Input: dimensioned drawing with shaded views. Units: mm. Origin: part minimum x, y, z. A direction names the side the tool comes from. Give positions to 0.01 mm unless a question says otherwise; leave off trailing zeros. Order: outer loops, then holes, each group sorted by start corner. A loop starts at its lowest first (then second) coordinate and runs counter-clockwise, first axis right, second up. Notation, with made-up numbers: M -0.75,88 L 7.25,88 A4 ccw 7.25,94 Z; hole C -27.5,0 d2. An arc over 180 degrees is marked long. Answer in a Markdown table with one row per item. Add a question column.
(1) Set-up query: the marked faces 4 and 5. Return all of +Z, -Z, +X, -X, +Y, -Y with unobstructed straight access to the full face (end or side cutting, diameter ignored); none if empty.
(2) Section query D-D, the plane y = 5. Return loops of the section in (x, z), plus the area to 3 significant figures.
(3) Section query A-A, the plane y = 29. Return loops of the section in (x, z).
(4) Section query B-B, the plane x = 11. Return loops of the section in (y, z).
(5) Material intervals for line 1 along X through (y, z) = (30.5, 7.5); line 2 along Z through (x, y) = (27, 51); line 3 along X through (y, z) = (46, 8), sorted ascending.
(6) Mould query, pull axis Y, two halves, no side actions, for the marked faces 1, 2 and 3. Classes: pulls with the +Y half, pulls with the -Y half, needs draft (parallel to the pull), parting line crosses it, or undercut.
(7) Section query C-C, the plane z = 8.25. Return loops of the section in (x, y) (3 decimals), plus the area to 3 significant figures.
(8) Pin query (flat end, axial travel): P1, Ø4, axis at y = 24, z = 5, coming from the +X side; P2, Ø2, axis at x = 35.5, y = 15, coming from the +Z side; P3, Ø1, axis at y = 22, z = 5.5, coming from the +X side; P4, Ø1.5, axis at x = 28.5, y = 46.5, coming from the -Z side. Return the tip coordinate at first contact, or that it passes through.
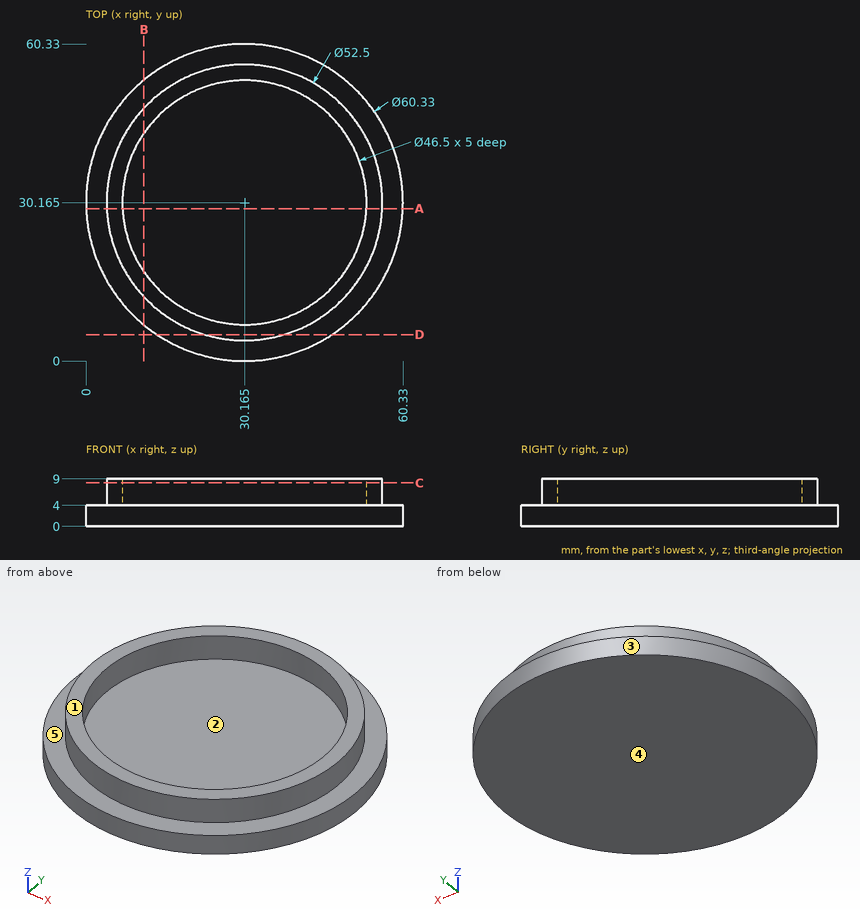
Values follow:
| question | item | result |
|---|---|---|
| 1 | face 4 | -Z, +X, -X, +Y, -Y |
| 1 | face 5 | +Z |
| 2 | outline | M 13.53,0 L 46.8,0 L 46.8,4 L 37.63,4 L 37.63,9 L 22.7,9 L 22.7,4 L 13.53,4 Z |
| 2 | area | 208 mm² |
| 3 | outline | M 0.02,0 L 60.31,0 L 60.31,4 L 56.39,4 L 56.39,9 L 53.39,9 L 53.39,4 L 6.94,4 L 6.94,9 L 3.94,9 L 3.94,4 L 0.02,4 Z |
| 4 | outline | M 6.87,0 L 53.46,0 L 53.46,4 L 48.1,4 L 48.1,9 L 43.33,9 L 43.33,4 L 17,4 L 17,9 L 12.23,9 L 12.23,4 L 6.87,4 Z |
| 5 | line 1 | x = 3.92 to 6.92, 53.41 to 56.41 |
| 5 | line 2 | z = 0 to 4 |
| 5 | line 3 | x = 9.23 to 13.14, 47.19 to 51.1 |
| 6 | face 1 | needs draft |
| 6 | face 2 | undercut |
| 6 | face 3 | parting line crosses it |
| 7 | outline | C 30.165,30.165 d52.5; hole C 30.165,30.165 d46.5 |
| 7 | area | 467 mm² |
| 8 | P1 | stops at x = 60 |
| 8 | P2 | stops at z = 4 |
| 8 | P3 | stops at x = 55.27 |
| 8 | P4 | stops at z = 0 |
